```python
from build123d import *

# Parameters (mm, degrees)
ESQUISSE1_W             = 40
ESQUISSE1_H             = 26
BOSS_EXTRU_1_DEPTH      = 15
ESQUISSE2_R             = 11
ENL_V_MAT_EXTRU_1_DEPTH = 7
ESQUISSE3_R             = 10
ENL_V_MAT_EXTRU_2_DEPTH = 1
ESQUISSE4_R             = 4.5
ENL_V_MAT_EXTRU_3_DEPTH = 7
ESQUISSE5_R             = 2.25
ENL_V_MAT_EXTRU_4_DEPTH = 51.009999


with BuildPart() as part:
    # Esquisse1 → Boss.-Extru.1 (new body)
    with BuildSketch(Plane.XY):
        with Locations((20, 13)):
            Rectangle(ESQUISSE1_W, ESQUISSE1_H)
    extrude(amount=BOSS_EXTRU_1_DEPTH)

    # Esquisse2 → Enlèv. mat.-Extru.1 (cut)
    with BuildSketch(Plane.XY.offset(15)):
        with Locations((20, 13)):
            Circle(ESQUISSE2_R)
    extrude(amount=-ENL_V_MAT_EXTRU_1_DEPTH, mode=Mode.SUBTRACT)

    # Esquisse3 → Enlèv. mat.-Extru.2 (cut)
    with BuildSketch(Plane.XY.offset(8)):
        with Locations((20, 13)):
            Circle(ESQUISSE3_R)
    extrude(amount=-ENL_V_MAT_EXTRU_2_DEPTH, mode=Mode.SUBTRACT)

    # Esquisse4 → Enlèv. mat.-Extru.3 (cut)
    with BuildSketch(Plane.XY.offset(7)):
        with Locations((20, 13)):
            Circle(ESQUISSE4_R)
    extrude(amount=-ENL_V_MAT_EXTRU_3_DEPTH, mode=Mode.SUBTRACT)

    # Esquisse5 → Enlèv. mat.-Extru.4 (cut, through all)
    with BuildSketch(Plane.XY.offset(15)):
        with Locations((5, 22)):
            Circle(ESQUISSE5_R)
        with Locations(Location((5, 4, 0), (0, 0, 180))):
            Circle(ESQUISSE5_R)
        with Locations((35, 4)):
            Circle(ESQUISSE5_R)
        with Locations(Location((35, 22, 0), (0, 0, 180))):
            Circle(ESQUISSE5_R)
    extrude(amount=-ENL_V_MAT_EXTRU_4_DEPTH, mode=Mode.SUBTRACT)


solid = part.part
```
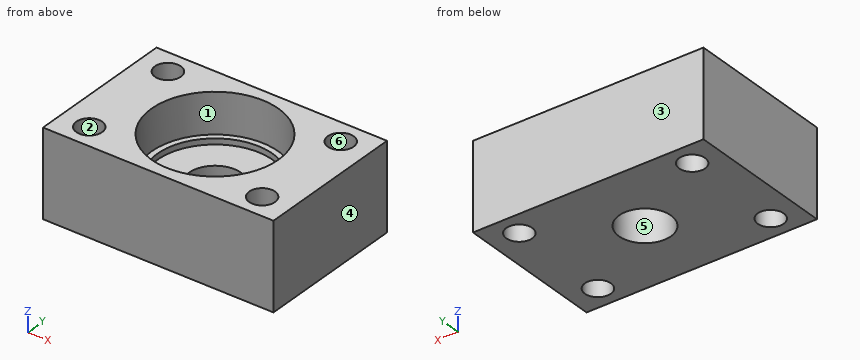
Here's how the part is built. I have some questions about the finished solid (model axes, mm). Face numbers are marked on the shaded views. A direction names the side the tool comes from. Give positions to 0.01 mm unless a question says otherwise; leave off trailing zeros. Write each loop counter-clockwise with the first axis right and the second up, starting at its lowest first coordinate (ties: lowest second). Pieces come first, ordered by that corner, then holes. Notation, with made-up numbers: (0.25, -36) -> (26.25, -36) arc R11 cw to (26.25, -26) -> close; hole circle Ø7 at (36.5, -7). An arc over 180 degrees is marked (long way). Use one line per item in the form item = value.
1) I'm going to push a flat-ended pin straight in: pin 1 (10.5 mm diameter, centred on x = 20, y = 13, fed in from +Z). Where does the tip first touch, or does it pass through?
Verdict:
pin_1 = 7
2) On a 3-axis mill with a long thin cutter (end or side, diameter ignored), from which of +Z, -Z, +X, -X, +Y, -Y can I reach the whole of each face in a straight line? I mean the marked faces 1 and 2. Say none if no direction works.
Verdict:
face_1 = +Z
face_2 = +Z, -Z
3) We'd pull the mould along X, two halves only. Please class the marked faces 3, 4, 5 and 6: +X half, -X half, draft (parallel to the pull), parting line (faces both ways), or undercut.
Verdict:
face_3 = draft
face_4 = +X half
face_5 = undercut
face_6 = undercut
4) Suppose I cut it at D-D (x = 20). Please give me the cut outline in (y, z).
Verdict:
outline = (0, 0) -> (8.5, 0) -> (8.5, 7) -> (3, 7) -> (3, 8) -> (2, 8) -> (2, 15) -> (0, 15) -> close; (17.5, 0) -> (26, 0) -> (26, 15) -> (24, 15) -> (24, 8) -> (23, 8) -> (23, 7) -> (17.5, 7) -> close
5) Suppose I cut it at C-C (z = 2.5). Please give me the cut outline in (x, y), and give its area (3 significant figures).
Verdict:
outline = (0, 0) -> (40, 0) -> (40, 26) -> (0, 26) -> close; hole circle Ø4.5 at (5, 4); hole circle Ø4.5 at (5, 22); hole circle Ø9 at (20, 13); hole circle Ø4.5 at (35, 4); hole circle Ø4.5 at (35, 22)
area = 913 mm2
6) Suppose I cut it at A-A (x = 35). Please give me the cut outline in (y, z).
Verdict:
outline = (0, 0) -> (1.75, 0) -> (1.75, 15) -> (0, 15) -> close; (6.25, 0) -> (19.75, 0) -> (19.75, 15) -> (6.25, 15) -> close; (24.25, 0) -> (26, 0) -> (26, 15) -> (24.25, 15) -> close
7) Suppose I cut it at B-B (y = 13). Please give me the cut outline in (x, z).
Verdict:
outline = (0, 0) -> (15.5, 0) -> (15.5, 7) -> (10, 7) -> (10, 8) -> (9, 8) -> (9, 15) -> (0, 15) -> close; (24.5, 0) -> (40, 0) -> (40, 15) -> (31, 15) -> (31, 8) -> (30, 8) -> (30, 7) -> (24.5, 7) -> close
8) If I drill on L1, parallel to Y at x = 5, z = 6.5; L2, parallel to X at y = 3.75, z = 8.75; L3, parallel to Y at x = 33, z = 0.5, over which ranges is the centre line in solid material (lowest first)? Write a range as [from, to].
Verdict:
L1 = [0, 1.75], [6.25, 19.75], [24.25, 26]
L2 = [0, 2.76], [7.24, 14.05], [25.95, 32.76], [37.24, 40]
L3 = [0, 2.97], [5.03, 20.97], [23.03, 26]
